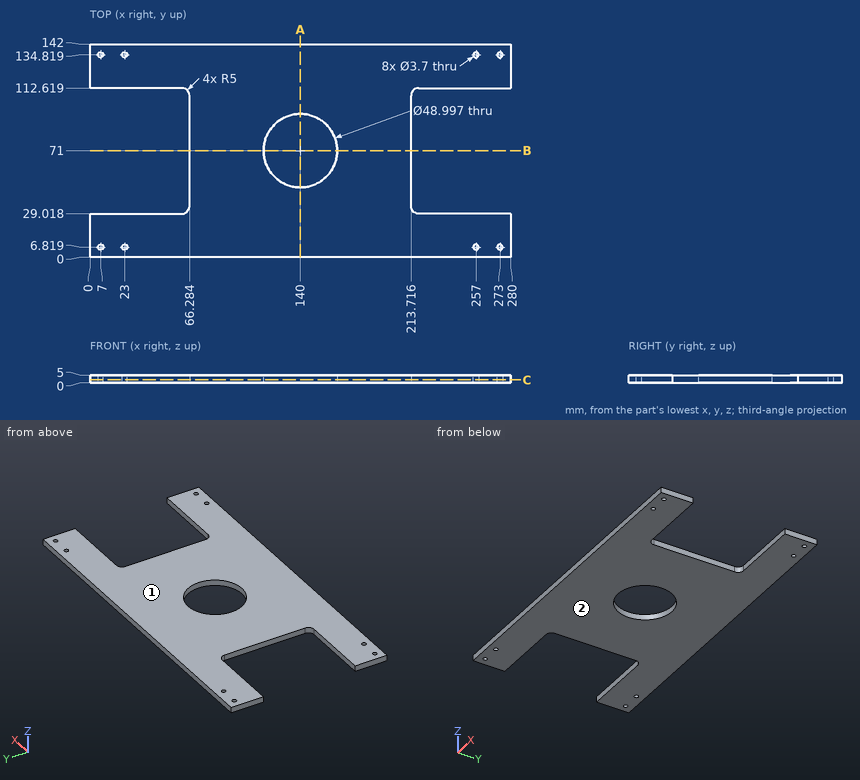
Answer from the drawing. Dimensions are ordinates in mm from the lowest x, y and z of the part. Coordinates: 2 decimals unless noted, no trailing zeros. Order: outer loops, then holes, each group sorted by start corner. A loop starts at its lowest first (then second) coordinate and runs counter-clockwise, first axis right, second up. Notation, with made-up numbers: M -24,89 L 26,89 A25 ccw 26,104 Z; hole C 28.5,-23 d8. An arc over 180 degrees is marked long. Put each result on its own line as item: value. Start each with the question number.
Item 1: Section B-B, the plane y = 71 is taken. Determine the outline of the cut face in (x, z).
Item 2: Section C-C, the plane z = 1.95 is taken. Count the separate pieces of the cut face and the enclosed holes in it, plus the area to 3 significant figures.
Item 3: Consider probe 1 along Y at (x, z) = (7, 3.2); probe 2 along Y at (x, z) = (140, 3.9); probe 3 along Y at (x, z) = (35, 1.75). Determine where each line is inside the solid, lowest interval first. Write a range as [from, to].
Item 4: Section A-A, the plane x = 140 is taken. Determine the outline of the cut face in (y, z).
Item 5: Given pin 1 Ø3 at (x, y) = (23, 134.82) entering from +Z, flat-ended and moving along its own axis, determine where the tip first touches the part or whether it passes through.
Item 6: The mould has two halves that part along Z. Classify the marked faces 1 and 2: +Z half, -Z half, draft (parallel to the pull), parting line (faces both ways), or undercut.
Computed:
1. outline: M 66.28,0 L 115.5,0 L 115.5,5 L 66.28,5 Z; M 164.5,0 L 213.72,0 L 213.72,5 L 164.5,5 Z
2. separate pieces: 1
2. enclosed holes: 9
2. area: 26,700 mm2
3. probe 1: y = [0, 4.97], [8.67, 29.02], [112.62, 132.97], [136.67, 142]
3. probe 2: y = [0, 46.5], [95.5, 142]
3. probe 3: y = [0, 29.02], [112.62, 142]
4. outline: M 0,0 L 46.5,0 L 46.5,5 L 0,5 Z; M 95.5,0 L 142,0 L 142,5 L 95.5,5 Z
5. pin 1: passes through
6. face 1: +Z half
6. face 2: -Z half
